```python
from build123d import *

# Parameters (mm, degrees)
SKETCH1_W           = 25.4
SKETCH1_H           = 63.5
SKETCH1_R           = 5.5245
BOSS_EXTRUDE1_DEPTH = 15.24
BOSS_EXTRUDE2_DEPTH = 63.5
SKETCH5_R           = 3.175
CUT_EXTRUDE3_DEPTH  = 138.137949616


with BuildPart() as part:
    # Sketch1 → Boss-Extrude1 (new body)
    with BuildSketch(Plane(origin=(0, 0, 0), x_dir=(1, 0, 0), z_dir=(0, 1, 0))):
        Rectangle(SKETCH1_W, SKETCH1_H)
        with Locations(Location((0, 0, 0), (0, 0, 90))):
            Circle(SKETCH1_R, mode=Mode.SUBTRACT)
    extrude(amount=BOSS_EXTRUDE1_DEPTH)

    # Sketch2 → Boss-Extrude2 (add)
    with BuildSketch(Plane.XY.offset(31.75)):
        Polygon((-9.525, 0), (-12.7, 0), (-12.7, -98.425), (-69.85, -98.425), (-69.85, -101.6), (-38.1, -101.6), (-9.525, -101.6), align=None)
    boss_extrude2 = extrude(amount=-BOSS_EXTRUDE2_DEPTH)

    # Mirror1: Boss-Extrude2 across plane
    add(boss_extrude2.mirror(Plane(origin=(0, 0, 0), x_dir=(0, 0, 1), z_dir=(1, 0, 0))))

    # Sketch5 → Cut-Extrude3 (cut, through all)
    with BuildSketch(Plane(origin=(0, -98.425, 0), x_dir=(1, 0, 0), z_dir=(0, 1, 0))):
        with Locations(Location((63.5, -25.4, 0), (0, 0, 180))):
            Circle(SKETCH5_R)
        with Locations(Location((50.8, -25.4, 0), (0, 0, 180))):
            Circle(SKETCH5_R)
        with Locations(Location((38.1, -25.4, 0), (0, 0, 180))):
            Circle(SKETCH5_R)
        with Locations(Location((25.4, -25.4, 0), (0, 0, 180))):
            Circle(SKETCH5_R)
        with Locations(Location((50.8, -12.7, 0), (0, 0, 180))):
            Circle(SKETCH5_R)
        with Locations(Location((38.1, -12.7, 0), (0, 0, 180))):
            Circle(SKETCH5_R)
        with Locations(Location((25.4, -12.7, 0), (0, 0, 180))):
            Circle(SKETCH5_R)
        with Locations(Location((50.8, 0, 0), (0, 0, 180))):
            Circle(SKETCH5_R)
        with Locations(Location((38.1, 0, 0), (0, 0, 180))):
            Circle(SKETCH5_R)
        with Locations(Location((25.4, 0, 0), (0, 0, 180))):
            Circle(SKETCH5_R)
        with Locations(Location((50.8, 12.7, 0), (0, 0, 180))):
            Circle(SKETCH5_R)
        with Locations(Location((38.1, 12.7, 0), (0, 0, 180))):
            Circle(SKETCH5_R)
        with Locations(Location((25.4, 12.7, 0), (0, 0, 180))):
            Circle(SKETCH5_R)
        with Locations(Location((50.8, 25.4, 0), (0, 0, 180))):
            Circle(SKETCH5_R)
        with Locations(Location((38.1, 25.4, 0), (0, 0, 180))):
            Circle(SKETCH5_R)
        with Locations(Location((25.4, 25.4, 0), (0, 0, 180))):
            Circle(SKETCH5_R)
        with Locations(Location((63.5, -12.7, 0), (0, 0, 180))):
            Circle(SKETCH5_R)
        with Locations(Location((63.5, 0, 0), (0, 0, 180))):
            Circle(SKETCH5_R)
        with Locations(Location((63.5, 12.7, 0), (0, 0, 180))):
            Circle(SKETCH5_R)
        with Locations(Location((63.5, 25.4, 0), (0, 0, 180))):
            Circle(SKETCH5_R)
        with Locations((-63.5, 25.4)):
            Circle(SKETCH5_R)
        with Locations((-63.5, 12.7)):
            Circle(SKETCH5_R)
        with Locations((-63.5, 0)):
            Circle(SKETCH5_R)
        with Locations((-63.5, -12.7)):
            Circle(SKETCH5_R)
        with Locations((-25.4, 25.4)):
            Circle(SKETCH5_R)
        with Locations((-38.1, 25.4)):
            Circle(SKETCH5_R)
        with Locations((-50.8, 25.4)):
            Circle(SKETCH5_R)
        with Locations((-25.4, 12.7)):
            Circle(SKETCH5_R)
        with Locations((-38.1, 12.7)):
            Circle(SKETCH5_R)
        with Locations((-50.8, 12.7)):
            Circle(SKETCH5_R)
        with Locations((-25.4, 0)):
            Circle(SKETCH5_R)
        with Locations((-38.1, 0)):
            Circle(SKETCH5_R)
        with Locations((-50.8, 0)):
            Circle(SKETCH5_R)
        with Locations((-25.4, -12.7)):
            Circle(SKETCH5_R)
        with Locations((-38.1, -12.7)):
            Circle(SKETCH5_R)
        with Locations((-50.8, -12.7)):
            Circle(SKETCH5_R)
        with Locations((-25.4, -25.4)):
            Circle(SKETCH5_R)
        with Locations((-38.1, -25.4)):
            Circle(SKETCH5_R)
        with Locations((-50.8, -25.4)):
            Circle(SKETCH5_R)
        with Locations((-63.5, -25.4)):
            Circle(SKETCH5_R)
    extrude(amount=-CUT_EXTRUDE3_DEPTH, mode=Mode.SUBTRACT)


solid = part.part
```
Read the model definition and answer for the solid it produces. Units are mm, in the model's axes. A direction names the side the tool comes from. Round coordinates to 2 decimals unless told otherwise and drop trailing zeros. Write each loop counter-clockwise with the first axis right and the second up, starting at its lowest first coordinate (ties: lowest second). Pieces come first, ordered by that corner, then holes. Notation, with made-up numbers: M -7,60 L 10,60 A22 cw 10,80 Z; hole C 28,-6 d2. An arc over 180 degrees is marked long. One line per item, written item: value.
Q1. Flat-ended cylindrical pins translate along their axes: pin 1 Ø7.5 at (x, z) = (25.4, 25.4) entering from +Y (3 decimals); pin 2 Ø5 at (x, z) = (50.8, -25.4) entering from +Y; pin 3 Ø8 at (y, z) = (-46.5, 6.5) entering from -X; pin 4 Ø1 at (y, z) = (-11.5, -16.5) entering from +X. Find the tip coordinate at first contact, or state that the pin passes through.
Data:
pin 1: y = -98.425
pin 2: through
pin 3: x = -12.7
pin 4: x = 12.7
Q2. Find section B-B on x = -38.1. Write down the section's boundary in (y, z) (3 decimals), plus the area to 3 significant figures.
Data:
outline: M -101.6,-31.75 L -98.425,-31.75 L -98.425,-28.575 L -101.6,-28.575 Z; M -101.6,-22.225 L -98.425,-22.225 L -98.425,-15.875 L -101.6,-15.875 Z; M -101.6,-9.525 L -98.425,-9.525 L -98.425,-3.175 L -101.6,-3.175 Z; M -101.6,3.175 L -98.425,3.175 L -98.425,9.525 L -101.6,9.525 Z; M -101.6,15.875 L -98.425,15.875 L -98.425,22.225 L -101.6,22.225 Z; M -101.6,28.575 L -98.425,28.575 L -98.425,31.75 L -101.6,31.75 Z
area: 101 mm2
Q3. Find section A-A on y = -25. Write down the section's boundary in (x, z) (3 decimals), plus the area to 3 significant figures.
Data:
outline: M -12.7,-31.75 L -9.525,-31.75 L -9.525,31.75 L -12.7,31.75 Z; M 9.525,-31.75 L 12.7,-31.75 L 12.7,31.75 L 9.525,31.75 Z
area: 403 mm2
Q4. Find section D-D on z = -25.4. Count the separate pieces of the cut face and the enclosed holes in it, plus the area to 3 significant figures.
Data:
separate pieces: 9
enclosed holes: 0
area: 1,230 mm2
Q5. Which of the six approach directions +Z, -Z, +X, -X, +Y, -Y give full straight-line access (tool end or side, diameter ignored) to faces 4 (the flat face through (6, 0, 0)), 5 (the flat face through (-34.5, -98.425, 0.4)), 6 (the cylindrical face through (53.97, -99.99, 0.14))?
Data:
face 4: +Z, -Z, -Y
face 5: +Z, -Z, -X, +Y
face 6: +Y, -Y
Q6. Straight lines are drawn through the part: line 1 (Z direction, x = -63.5, y = -99.9) (3 decimals); line 2 (Z direction, x = -25, y = -100); line 3 (X direction, y = -14, z = 2.5) (3 decimals). For each, find the intervals that lie inside material, in ascending order. Write a range as [from, to].
Data:
line 1: [-31.75, -28.575], [-22.225, -15.875], [-9.525, -3.175], [3.175, 9.525], [15.875, 22.225], [28.575, 31.75]
line 2: [-31.75, -28.55], [-22.25, -15.85], [-9.55, -3.15], [3.15, 9.55], [15.85, 22.25], [28.55, 31.75]
line 3: [-12.7, -9.525], [9.525, 12.7]
Q7. For a pull along X with two mould halves and no side action, classify faces 1 (the cylindrical face through (-40.44, -99.99, -27.546)), 2 (the flat face through (-10, -52, 31.75)), 3 (the flat face through (-12.7, -41, 0)) as +X half, -X half, draft (parallel to the pull), parting line (faces both ways), or undercut.
Data:
face 1: undercut
face 2: draft
face 3: -X half
Q8. Find section C-C on y = 8.5. Write down the section's boundary in (x, z), plus the area to 3 significant figures.
Data:
outline: M -12.7,-31.75 L 12.7,-31.75 L 12.7,31.75 L -12.7,31.75 Z; hole C 0,0 d11.05
area: 1,520 mm2
